Input: dimensioned drawing with shaded views. Units: mm. Origin: part minimum x, y, z. A direction names the side the tool comes from. Round coordinates to 2 decimals unless told otherwise and drop trailing zeros. Loops run counter-clockwise (first coordinate to the right, second up) from the corner with the lowest first, then second, coordinate; pieces in that order, holes last.
1) Section A-A, the plane y = 12.5. Return loops of the section in (x, z) (1 decimal), and give its area (3 significant figures).
2) Section C-C, the plane x = 13.5. Return loops of the section in (y, z) (1 decimal).
3) Ray query, line 1 along X through (y, z) = (2.75, 11.75); line 2 along X through (y, z) = (13, 5.5); line 3 along Z through (x, y) = (6.5, 13.5). Return the intervals inside material, ascending.
4) Section D-D, the plane z = 19. Return loops of the section in (x, y) (1 decimal).
5) Section B-B, the plane z = 7.75. Return loops of the section in (x, y), and give its area (3 significant figures).
6) First-contact query: pin 1 (10 mm diameter, centred on y = 18.5, z = 22.5, fed in from +X); pin 2 (1 mm diameter, centred on y = 7.5, z = 4, fed in from -X); pin 3 (12.5 mm diameter, centred on y = 8.5, z = 7, fed in from +X); pin 4 (2 mm diameter, centred on x = 14.5, y = 10, fed in from +Z). Flat tips, straight axial feed; report the tip coordinate or a pass-through.
7) Access query for the marked faces 1, 2 and 3. Directions: +Z, -Z, +X, -X, +Y, -Y. A direction counts if a zero-diameter tool reaches every point of the face in a straight line with its end or side. Return the directions, or none.
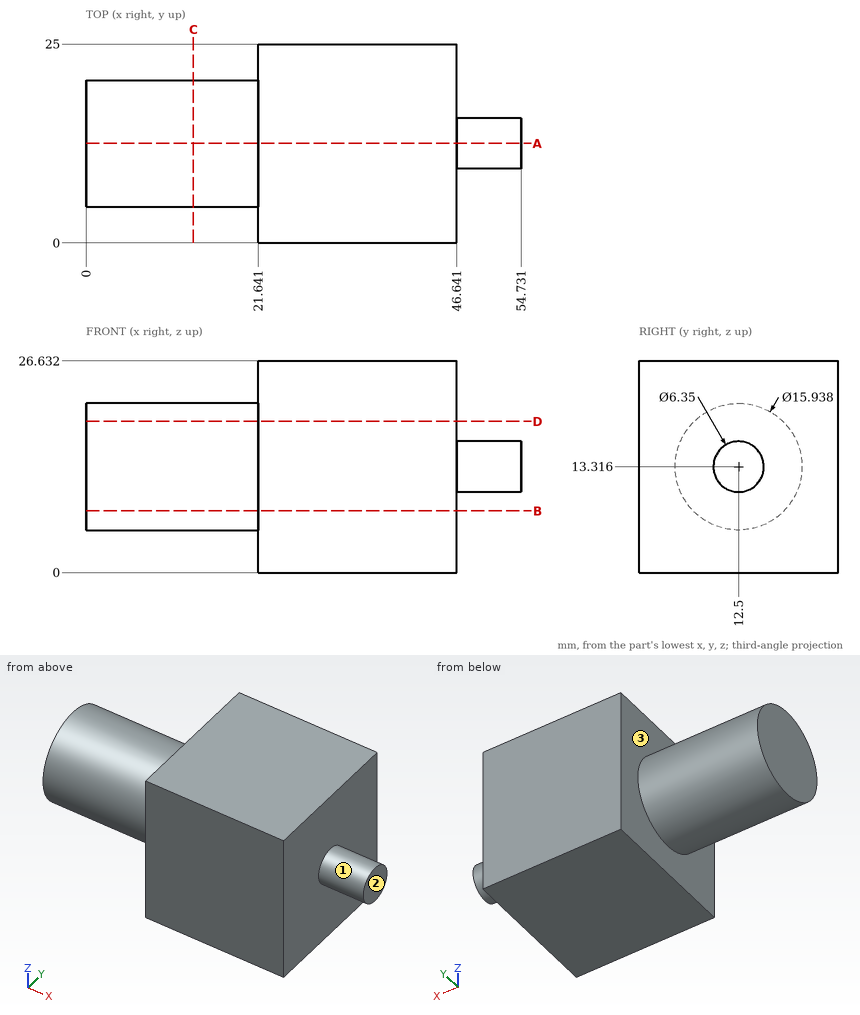
Final values:
1. outline: (0, 5.3) - (21.6, 5.3) - (21.6, 0) - (46.6, 0) - (46.6, 10.1) - (54.7, 10.1) - (54.7, 16.5) - (46.6, 16.5) - (46.6, 26.6) - (21.6, 26.6) - (21.6, 21.3) - (0, 21.3) - close
1. area: 1,060 mm2
2. outline: circle Ø15.9 at (12.5, 13.3)
3. line 1: x = 21.64 to 46.64
3. line 2: x = 0 to 46.64
3. line 3: z = 5.41 to 21.22
4. outline: (0, 6.9) - (21.6, 6.9) - (21.6, 0) - (46.6, 0) - (46.6, 25) - (21.6, 25) - (21.6, 18.1) - (0, 18.1) - close
5. outline: (0, 6.8) - (21.64, 6.8) - (21.64, 0) - (46.64, 0) - (46.64, 25) - (21.64, 25) - (21.64, 18.2) - (0, 18.2) - close
5. area: 872 mm2
6. pin 1: stops at x = 46.64
6. pin 2: stops at x = 21.64
6. pin 3: stops at x = 54.73
6. pin 4: stops at z = 21.14
7. face 1: +X
7. face 2: +Z, -Z, +X, +Y, -Y
7. face 3: -X
